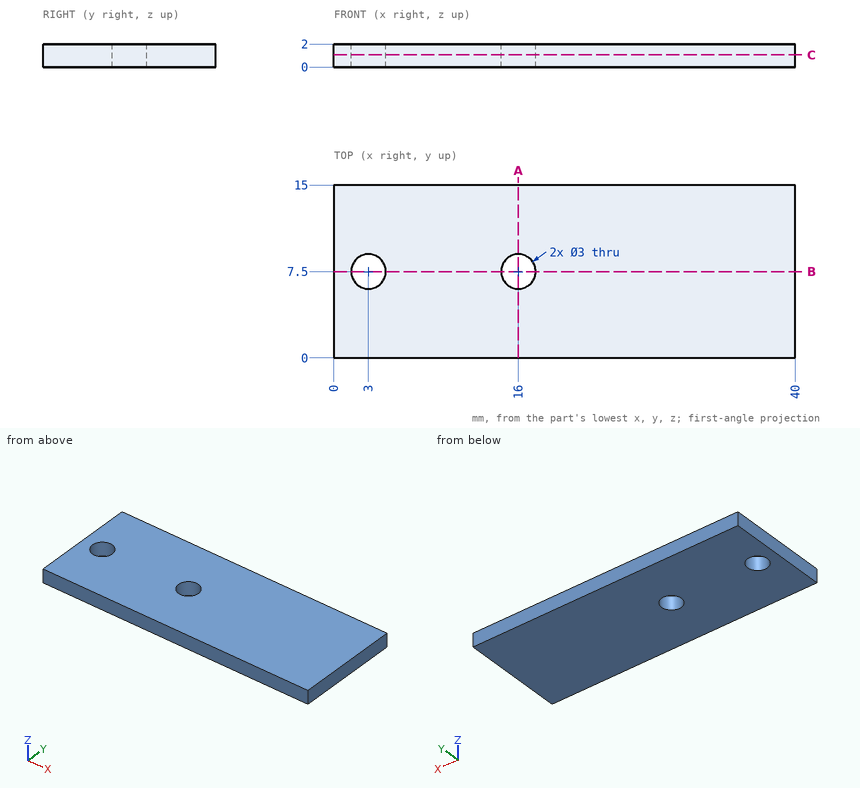
Design review of the part shown in the three views and the two pictorial views. Dimensions are in mm from the part's minimum x, y and z. Round coordinates to 2 decimals unless told otherwise and drop trailing zeros. Loops run counter-clockwise (first coordinate to the right, second up) from the corner with the lowest first, then second, coordinate; pieces in that order, holes last. Notation, with made-up numbers: (62.5, 64.5) - (104.5, 64.5) arc R33 cw to (104.5, 93.5) - close; hole circle Ø5 at (-10.5, 78.25). An arc over 180 degrees is marked (long way). One line per item, written item: value. Start each with the question number.
Item 1: For L1, parallel to X at y = 7.5, z = 1.5; L2, parallel to Y at x = 3, z = 1.45, list the stretches that pass through material, from the lowest coordinate up.
Item 2: Take a section at C-C (z = 1.05). Give the boundary of the cut face in (x, y), plus the area to 3 significant figures.
Item 3: Take a section at A-A (x = 16). Give the boundary of the cut face in (y, z), plus the area to 3 significant figures.
Item 4: Take a section at B-B (y = 7.5). Give the boundary of the cut face in (x, z).
Answer below:
1. L1: x = 0 to 1.5, 4.5 to 14.5, 17.5 to 40
1. L2: y = 0 to 6, 9 to 15
2. outline: (0, 0) - (40, 0) - (40, 15) - (0, 15) - close; hole circle Ø3 at (3, 7.5); hole circle Ø3 at (16, 7.5)
2. area: 586 mm2
3. outline: (0, 0) - (6, 0) - (6, 2) - (0, 2) - close; (9, 0) - (15, 0) - (15, 2) - (9, 2) - close
3. area: 24.0 mm2
4. outline: (0, 0) - (1.5, 0) - (1.5, 2) - (0, 2) - close; (4.5, 0) - (14.5, 0) - (14.5, 2) - (4.5, 2) - close; (17.5, 0) - (40, 0) - (40, 2) - (17.5, 2) - close
